from build123d import *

# Parameters (mm, degrees)
SKETCH_1_R           = 1.5
EXTRUDE_1_DEPTH      = 1.6
EXTRUDE_2_DEPTH      = 5.6
SKETCH_3_R           = 6
SKETCH_3_R_2         = 5
EXTRUDE_3_DEPTH      = 7.6
SKETCH_4_R           = 3.5
SKETCH_4_R_2         = 2.75
EXTRUDE_4_DEPTH      = 9.6
SKETCH_5_R           = 3.5
EXTRUDE_5_DEPTH      = 9.6
EXTRUDE_6_DEPTH      = 0.001
EXTRUDE_6_DEPTH_BACK = 1.1
SKETCH_7_W           = 12
SKETCH_7_H           = 4.716784086


with BuildPart() as part:
    # 草图1 → 凸台-拉伸1 (new body)
    with BuildSketch(Plane(origin=(0, 0, 0), x_dir=(1, 0, 0), z_dir=(0, 1, 0))):
        with BuildLine():
            Line((-9.5, 11.022466342), (9.5, 11.022466342))
            ThreePointArc((9.5, 11.022466342), (14.449747468, 8.97221381), (16.5, 4.022466342))
            Line((16.5, 4.022466342), (16.5, -7.977533658))
            ThreePointArc((16.5, -7.977533658), (13.571067812, -15.04860147), (6.5, -17.977533658))
            Line((6.5, -17.977533658), (-6.5, -17.977533658))
            ThreePointArc((-6.5, -17.977533658), (-13.571067812, -15.04860147), (-16.5, -7.977533658))
            Line((-16.5, -7.977533658), (-16.5, 4.022466342))
            ThreePointArc((-16.5, 4.022466342), (-14.449747468, 8.97221381), (-9.5, 11.022466342))
        make_face()
        with Locations(Location((-13.3, 6, 0), (0, 0, 270))):
            Circle(SKETCH_1_R, mode=Mode.SUBTRACT)
        with Locations(Location((13.3, 6, 0), (0, 0, 270))):
            Circle(SKETCH_1_R, mode=Mode.SUBTRACT)
        with Locations(Location((-13.3, -6, 0), (0, 0, 270))):
            Circle(SKETCH_1_R, mode=Mode.SUBTRACT)
        with Locations(Location((13.3, -6, 0), (0, 0, 270))):
            Circle(SKETCH_1_R, mode=Mode.SUBTRACT)
        with BuildLine():
            Line((-11, 0.75), (-10, 0.75))
            ThreePointArc((-10, 0.75), (-9.25, 0), (-10, -0.75))
            Line((-10, -0.75), (-11, -0.75))
            ThreePointArc((-11, -0.75), (-11.75, 0), (-11, 0.75))
        make_face(mode=Mode.SUBTRACT)
        with BuildLine():
            Line((11, 0.75), (10, 0.75))
            ThreePointArc((10, 0.75), (9.25, 0), (10, -0.75))
            Line((10, -0.75), (11, -0.75))
            ThreePointArc((11, -0.75), (11.75, 0), (11, 0.75))
        make_face(mode=Mode.SUBTRACT)
    extrude(amount=EXTRUDE_1_DEPTH)

    # 草图2 → 凸台-拉伸2 (add)
    with BuildSketch(Plane(origin=(0, 0, 0), x_dir=(1, 0, 0), z_dir=(0, 1, 0))):
        with BuildLine():
            Line((-7.5, 8.022466342), (7.5, 8.022466342))
            ThreePointArc((7.5, 8.022466342), (9.621320344, 7.143786685), (10.5, 5.022466342))
            Line((10.5, 5.022466342), (10.5, -6.977533658))
            ThreePointArc((10.5, -6.977533658), (9.621320344, -9.098854002), (7.5, -9.977533658))
            Line((7.5, -9.977533658), (-7.5, -9.977533658))
            ThreePointArc((-7.5, -9.977533658), (-9.621320344, -9.098854002), (-10.5, -6.977533658))
            Line((-10.5, -6.977533658), (-10.5, 5.022466342))
            ThreePointArc((-10.5, 5.022466342), (-9.621320344, 7.143786685), (-7.5, 8.022466342))
        make_face()
    extrude(amount=EXTRUDE_2_DEPTH)

    # 草图3 → 凸台-拉伸3 (add)
    with BuildSketch(Plane(origin=(0, 0, 0), x_dir=(1, 0, 0), z_dir=(0, 1, 0))):
        with Locations(Location((0, 0, 0), (0, 0, 90))):
            Circle(SKETCH_3_R)
        with Locations(Location((0, 0, 0), (0, 0, 90))):
            Circle(SKETCH_3_R_2, mode=Mode.SUBTRACT)
    extrude(amount=EXTRUDE_3_DEPTH)

    # 草图4 → 凸台-拉伸4 (add)
    with BuildSketch(Plane(origin=(0, 0, 0), x_dir=(1, 0, 0), z_dir=(0, 1, 0))):
        with Locations(Location((0, 0, 0), (0, 0, 270))):
            Circle(SKETCH_4_R)
        with Locations(Location((0, 0, 0), (0, 0, 270))):
            Circle(SKETCH_4_R_2, mode=Mode.SUBTRACT)
    extrude(amount=EXTRUDE_4_DEPTH)

    # 草图5 → 凸台-拉伸5 (add)
    with BuildSketch(Plane(origin=(0, 0, 0), x_dir=(1, 0, 0), z_dir=(0, 1, 0))):
        with Locations(Location((0, 0, 0), (0, 0, 270))):
            Circle(SKETCH_5_R)
    extrude(amount=EXTRUDE_5_DEPTH)

    # 草图7 → 凸台-拉伸6 (add, two sides: drawn at the far end of the back side and taken through both)
    with BuildSketch(Plane(origin=(0, 0, 0), x_dir=(1, 0, 0), z_dir=(0, 1, 0)).offset(-EXTRUDE_6_DEPTH_BACK)):
        with Locations((0, -15.619141615)):
            Rectangle(SKETCH_7_W, SKETCH_7_H)
    extrude(amount=EXTRUDE_6_DEPTH + EXTRUDE_6_DEPTH_BACK)


solid = part.part
The model under review builds one solid part; all positions refer to its coordinate system, in mm. A direction names the side the tool comes from. Round coordinates to 2 decimals unless told otherwise and drop trailing zeros. Loops run counter-clockwise (first coordinate to the right, second up) from the corner with the lowest first, then second, coordinate; pieces in that order, holes last. Notation, with made-up numbers: M 8.5,-26 L 60.5,-26 A9 cw 60.5,-20 Z; hole C -17,8 d4. An arc over 180 degrees is marked long. Answer as CSV lines item,"result". Start each with the question number.
Item 1: Mouldability with a two-part tool opening along X and no side actions: class faces 6 (the face through (0, 1, -11.022)), 7 (the face through (9.598, 3.572, -7.167)), 8 (the face through (11.75, 0.79, 0.02)) as released by +X, released by -X, zero draft, split by the parting line, or undercut.
Item 2: Insertion check: P1, Ø1.8, axis at x = 13.3, z = 6, coming from the -Y side; P2, Ø1.7, axis at y = 3, z = 3, coming from the -X side; P3, Ø4, axis at x = 13.3, z = -6, coming from the -Y side; P4, Ø2, axis at x = 3.5, y = 3.5, coming from the +Z side. Each pin has a flat end and moves straight along its axis. Give the tip position at first contact, or say it passes through.
Item 3: For faces 1 (the face through (-9.6, 3.57, 9.12)), 2 (the face through (-0.1, -0.6, 13.261)), 3 (the face through (-9.645, 3.572, -7.12)), 4 (the face through (-2.2, 5.6, 3.3)), 5 (the face through (0, 4, -8.022)), list the 3-axis set-ups (+Z, -Z, +X, -X, +Y, -Y) from which the entire face can be reached by the end or side of a thin tool; tool diameter is ignored.
Item 4: Consider section D-D (x = 8). Write out the cut boundary in (y, z).
Item 5: Wall thickness on line 1 (X direction, y = 6.55, z = 0); line 2 (X direction, y = 1, z = 6); line 3 (X direction, y = 2.25, z = -1): over which ranges is each line inside the solid? List them lowest first. Write a range as [from, to].
Item 6: Consider section A-A (z = 0). Write out the cut boundary in (x, y), then the cut area to 3 significant figures.
Item 7: Consider section C-C (y = 7). Write out the cut boundary in (x, z).
Item 8: Consider section B-B (x = 12.5). Write out the cut boundary in (y, z), then the cut area to 3 significant figures.
Answer:
1,face 6,"zero draft"
1,face 7,"released by +X"
1,face 8,"undercut"
2,P1,"passes through"
2,P2,"stops at x = -10.5"
2,P3,"stops at y = 0"
2,P4,"stops at z = 9.98"
3,face 1,"+Z, -X, +Y"
3,face 2,"-Z, +X, -X, -Y"
3,face 3,"-Z, -X, +Y"
3,face 4,"+Y"
3,face 5,"-Z, +X, -X, +Y"
4,outline,"M 0,-11.02 L 1.6,-11.02 L 1.6,-7.98 L 5.6,-7.98 L 5.6,9.94 L 1.6,9.94 L 1.6,17.86 L 0,17.86 Z"
5,line 1,"x = [-6, -5], [-3.5, 3.5], [5, 6]"
5,line 2,"x = [-16.5, -14.8], [-11.8, 11.8], [14.8, 16.5]"
5,line 3,"x = [-10.5, 10.5]"
6,outline,"M -16.5,0 L -11.75,0 L -11.75,1.6 L -16.5,1.6 Z; M -10.5,0 L 10.5,0 L 10.5,5.6 L 6,5.6 L 6,7.6 L 5,7.6 L 5,5.6 L 3.5,5.6 L 3.5,9.6 L -3.5,9.6 L -3.5,5.6 L -5,5.6 L -5,7.6 L -6,7.6 L -6,5.6 L -10.5,5.6 Z; M 11.75,0 L 16.5,0 L 16.5,1.6 L 11.75,1.6 Z"
6,area,"165 mm^2"
7,outline,"C 0,0 d12; C 0,0 d7; hole C 0,0 d10"
8,outline,"M 0,-10.35 L 1.6,-10.35 L 1.6,-7.27 L 0,-7.27 Z; M 0,-4.73 L 1.6,-4.73 L 1.6,4.73 L 0,4.73 Z; M 0,7.27 L 1.6,7.27 L 1.6,15.98 L 0,15.98 Z"
8,area,"34.0 mm^2"
